Source: CAD feature listing. Evaluate the final solid. Frame: model axes, mm. A direction names the side the tool comes from. Give positions to 0.01 mm unless a question says otherwise; leave off trailing zeros. Loops run counter-clockwise (first coordinate to the right, second up) from the corner with the lowest first, then second, coordinate; pieces in that order, holes last. Notation, with made-up numbers: M 82,87 L 101,87 A15 ccw 101,115 Z; hole C 4.5,76.5 d11. An arc over 180 degrees is marked long. Write item = value, one per line.
from build123d import *

# Parameters (mm, degrees)
SKETCH_1_W          = 16
SKETCH_1_H          = 30
SKETCH_1_R          = 1.75
EXTRUDE_3_DEPTH     = 4
SKETCH_4_W          = 16
SKETCH_4_H          = 8
EXTRUDE_4_DEPTH     = 38
SKETCH_6_R          = 1.5
CUT_EXTRUDE_1_DEPTH = 10


with BuildPart() as part:
    # 草图1 → 凸台-拉伸3 (new body)
    with BuildSketch(Plane.XY):
        Rectangle(SKETCH_1_W, SKETCH_1_H)
        with Locations((-5, 7.5)):
            Circle(SKETCH_1_R, mode=Mode.SUBTRACT)
        with Locations(Location((5, 7.5, 0), (0, 0, 180))):
            Circle(SKETCH_1_R, mode=Mode.SUBTRACT)
        with Locations((5, -7.5)):
            Circle(SKETCH_1_R, mode=Mode.SUBTRACT)
        with Locations(Location((-5, -7.5, 0), (0, 0, 180))):
            Circle(SKETCH_1_R, mode=Mode.SUBTRACT)
    extrude(amount=EXTRUDE_3_DEPTH)

    # 草图4 → 凸台-拉伸4 (add)
    with BuildSketch(Plane.XY.offset(4)):
        Rectangle(SKETCH_4_W, SKETCH_4_H)
    extrude(amount=EXTRUDE_4_DEPTH)

    # 草图6 → 切除-拉伸1 (cut)
    with BuildSketch(Plane.XY.offset(42)):
        with Locations((-4, 0)):
            Circle(SKETCH_6_R)
        with Locations(Location((4, 0, 0), (0, 0, 180))):
            Circle(SKETCH_6_R)
    extrude(amount=-CUT_EXTRUDE_1_DEPTH, mode=Mode.SUBTRACT)


solid = part.part
1. Reachability of faces 1 (the cylindrical face through (-2.614, -0.575, 37.07)), 2 (the flat face through (0, 10, 4)), 3 (the flat face through (0, -9, 4)), 4 (the cylindrical face through (3.61, -8.56, 1.97)) from +Z, -Z, +X, -X, +Y, -Y: full face, straight path, thin tool, end or side. Return the list, or none.
Derived:
face_1 = +Z
face_2 = +Z, +X, -X, +Y
face_3 = +Z, +X, -X, -Y
face_4 = +Z, -Z
2. First-contact query: pin 1 Ø1 at (x, z) = (0.5, 37) entering from -Y; pin 2 Ø5 at (x, z) = (-0.5, 24) entering from +Y; pin 3 Ø4 at (x, y) = (-5, -7.5) entering from +Z. Flat tips, straight axial feed; report the tip coordinate or a pass-through.
Derived:
pin_1 = -4
pin_2 = 4
pin_3 = 4
3. Cut plane B-B, the plane x = 5. Return the cut outline in (y, z).
Derived:
outline = M -15,0 L -9.25,0 L -9.25,4 L -15,4 Z; M -5.75,0 L 5.75,0 L 5.75,4 L 4,4 L 4,42 L 1.12,42 L 1.12,32 L -1.12,32 L -1.12,42 L -4,42 L -4,4 L -5.75,4 Z; M 9.25,0 L 15,0 L 15,4 L 9.25,4 Z
4. Pull-direction query (X, two-part tool) for faces 5 (the flat face through (4, 0, 32)), 6 (the cylindrical face through (-3.25, -7.58, 1.97)), 7 (the flat face through (-8, 0, 16)), 8 (the flat face through (0, -4, 23)); classes: +X half, -X half, draft (parallel to the pull), parting line (faces both ways), or undercut.
Derived:
face_5 = undercut
face_6 = undercut
face_7 = -X half
face_8 = draft
5. Material intervals for probe 1 along Y at (x, z) = (-5, 2.55); probe 2 along Y at (x, z) = (4, 35.75); probe 3 along Z at (x, y) = (7, -12.25), sorted ascending. Write a range as from..to.
Derived:
probe_1 = -15..-9.25, -5.75..5.75, 9.25..15
probe_2 = -4..-1.5, 1.5..4
probe_3 = 0..4
6. Cut plane D-D, the plane z = 8. Return the cut outline in (x, y), then the cut area to 3 significant figures.
Derived:
outline = M -8,-4 L 8,-4 L 8,4 L -8,4 Z
area = 128 mm²
7. Cut plane A-A, the plane y = 7.5. Return the cut outline in (x, z), then the cut area to 3 significant figures.
Derived:
outline = M -8,0 L -6.75,0 L -6.75,4 L -8,4 Z; M -3.25,0 L 3.25,0 L 3.25,4 L -3.25,4 Z; M 6.75,0 L 8,0 L 8,4 L 6.75,4 Z
area = 36.0 mm²
8. Cut plane C-C, the plane z = 34.5. Return the cut outline in (x, y).
Derived:
outline = M -8,-4 L 8,-4 L 8,4 L -8,4 Z; hole C -4,0 d3; hole C 4,0 d3
